Can you work these out from the drawing? Everything is in mm from the part's minimum corner. A direction names the side the tool comes from. Round coordinates to 2 decimals unless told otherwise and drop trailing zeros. Order: outer loops, then holes, each group sorted by start corner. A loop starts at its lowest first (then second) coordinate and runs counter-clockwise, first axis right, second up. Notation, with made-up numbers: (38, -30.5) - (65, -30.5) arc R22 ccw to (65, -12.5) - close; hole circle Ø8 at (54, -9). An arc over 180 degrees is marked (long way). Write item = value, one per line.
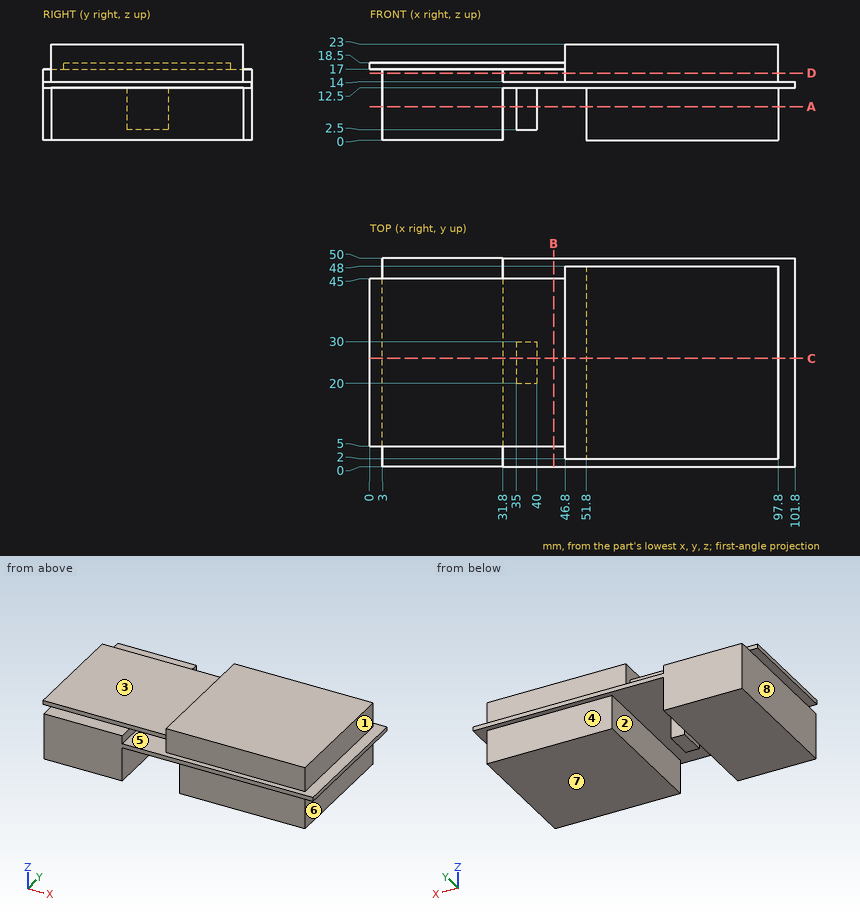
(1) If I drill on line 1 (X direction, y = 28, z = 5); line 2 (X direction, y = 37, z = 4); line 3 (X direction, y = 12.5, z = 14.75), over which ranges is the centre line in solid material (lowest first)? Write a range as from..to.
Computed:
line_1 = 3..31.8, 35..40, 51.8..97.8
line_2 = 3..31.8, 51.8..97.8
line_3 = 3..31.8, 46.8..97.8
(2) If we section it at B-B (x = 44): Write out the boundary of the cut face in (y, z).
Computed:
outline = (0, 12.5) - (50, 12.5) - (50, 14) - (0, 14) - close; (5, 17) - (45, 17) - (45, 18.5) - (5, 18.5) - close
(3) Thinking about a two-plate mould opening in X: for the marked faces 5, 6, 7 and 8, which applies, +X half, -X half, draft (parallel to the pull), parting line (faces both ways), or undercut?
Computed:
face_5 = undercut
face_6 = +X half
face_7 = draft
face_8 = -X half
(4) If we section it at C-C (y = 26): Write out the boundary of the cut face in (x, z), plus the area to 3 significant figures.
Computed:
outline = (0, 17) - (3, 17) - (3, 0) - (31.8, 0) - (31.8, 12.5) - (35, 12.5) - (35, 2.5) - (40, 2.5) - (40, 12.5) - (51.8, 12.5) - (51.8, 0) - (97.8, 0) - (97.8, 12.5) - (101.8, 12.5) - (101.8, 14) - (97.8, 14) - (97.8, 23) - (46.8, 23) - (46.8, 18.5) - (0, 18.5) - close; hole (31.8, 14) - (46.8, 14) - (46.8, 17) - (31.8, 17) - close
area = 1,750 mm^2
(5) Will these pins go through, and if not, where does the flat tip stop? P1, Ø7, axis at x = 84.5, z = 19.5, coming from the +Y side; P2, Ø12, axis at x = 31, y = 17, coming from the +Z side; P3, Ø15, axis at x = 60.5, y = 36, coming from the -Z side; P4, Ø1.5, axis at x = 38, z = 10, coming from the +Y side.
Computed:
P1 = 48
P2 = 18.5
P3 = 0
P4 = 30
(6) If we section it at A-A (z = 8): Write out the boundary of the cut face in (x, y).
Computed:
outline = (3, 0) - (31.8, 0) - (31.8, 50) - (3, 50) - close; (35, 20) - (40, 20) - (40, 30) - (35, 30) - close; (51.8, 2) - (97.8, 2) - (97.8, 48) - (51.8, 48) - close
(7) If we section it at D-D (z = 16): Write out the boundary of the cut face in (x, y).
Computed:
outline = (3, 0) - (31.8, 0) - (31.8, 50) - (3, 50) - close; (46.8, 2) - (97.8, 2) - (97.8, 48) - (46.8, 48) - close
(8) On a 3-axis mill with a long thin cutter (end or side, diameter ignored), from which of +Z, -Z, +X, -X, +Y, -Y can I reach the whole of each face in a straight line? I mean the marked faces 1, 2, 3 and 4. Say none if no direction works.
Computed:
face_1 = +Z, +X, +Y, -Y
face_2 = -Z, +Y, -Y
face_3 = +Z, -X, +Y, -Y
face_4 = -Z, +X, +Y
